```python
from build123d import *

# Parameters (mm, degrees)
F0_R     = 3.25
F0_R_2   = 1.85
F1_DEPTH = 4
F2_DEPTH = 4
F3_R     = 2.54


with BuildPart() as f1:
    # F0 (on Top) → F1 (new body)
    with BuildSketch(Plane.XY):
        with BuildLine():
            ThreePointArc((16, 9.294458), (9.088031, 9.088031), (9.294458, 16))
            Line((9.294458, 16), (-9.294458, 16))
            ThreePointArc((-9.294458, 16), (-8.114579, 14.394727), (-7.696788, 12.446788))
            ThreePointArc((-7.696788, 12.446788), (-10.760855, 8.006053), (-16, 9.294458))
            Line((-16, 9.294458), (-16, -9.294458))
            ThreePointArc((-16, -9.294458), (-10.760855, -8.006053), (-7.696788, -12.446788))
            ThreePointArc((-7.696788, -12.446788), (-8.114579, -14.394727), (-9.294458, -16))
            Line((-9.294458, -16), (9.294458, -16))
            ThreePointArc((9.294458, -16), (9.088031, -9.088031), (16, -9.294458))
            Line((16, -9.294458), (16, 9.294458))
        make_face()
        with Locations((-6.363961, -6.363961)):
            Circle(F0_R, mode=Mode.SUBTRACT)
        with Locations((6.363961, -6.363961)):
            Circle(F0_R, mode=Mode.SUBTRACT)
        with Locations((-6.363961, 6.363961)):
            Circle(F0_R, mode=Mode.SUBTRACT)
        with Locations((6.363961, 6.363961)):
            Circle(F0_R, mode=Mode.SUBTRACT)
        with BuildLine():
            ThreePointArc((-7.696788, 12.446788), (-8.114579, 14.394727), (-9.294458, 16))
            Line((-9.294458, 16), (-15.599119, 16))
            ThreePointArc((-15.599119, 16), (-15.805546, 15.805546), (-16, 15.599119))
            Line((-16, 15.599119), (-16, 9.294458))
            ThreePointArc((-16, 9.294458), (-10.760855, 8.006053), (-7.696788, 12.446788))
        make_face()
        with Locations((-12.446788, 12.446788)):
            Circle(F0_R_2, mode=Mode.SUBTRACT)
        with BuildLine():
            ThreePointArc((16, 15.599119), (15.805546, 15.805546), (15.599119, 16))
            Line((15.599119, 16), (9.294458, 16))
            ThreePointArc((9.294458, 16), (9.088031, 9.088031), (16, 9.294458))
            Line((16, 9.294458), (16, 15.599119))
        make_face()
        with Locations((12.446788, 12.446788)):
            Circle(F0_R_2, mode=Mode.SUBTRACT)
        with BuildLine():
            Line((16, -15.599119), (16, -9.294458))
            ThreePointArc((16, -9.294458), (9.088031, -9.088031), (9.294458, -16))
            Line((9.294458, -16), (15.599119, -16))
            ThreePointArc((15.599119, -16), (15.805546, -15.805546), (16, -15.599119))
        make_face()
        with Locations((12.446788, -12.446788)):
            Circle(F0_R_2, mode=Mode.SUBTRACT)
        with BuildLine():
            Line((-15.599119, -16), (-9.294458, -16))
            ThreePointArc((-9.294458, -16), (-8.114579, -14.394727), (-7.696788, -12.446788))
            ThreePointArc((-7.696788, -12.446788), (-10.760855, -8.006053), (-16, -9.294458))
            Line((-16, -9.294458), (-16, -15.599119))
            ThreePointArc((-16, -15.599119), (-15.805546, -15.805546), (-15.599119, -16))
        make_face()
        with Locations((-12.446788, -12.446788)):
            Circle(F0_R_2, mode=Mode.SUBTRACT)
        with BuildLine():
            ThreePointArc((-16, 15.599119), (-15.805546, 15.805546), (-15.599119, 16))
            Line((-15.599119, 16), (-16, 16))
            Line((-16, 16), (-16, 15.599119))
        make_face()
        with BuildLine():
            Line((16, 15.599119), (16, 16))
            Line((16, 16), (15.599119, 16))
            ThreePointArc((15.599119, 16), (15.805546, 15.805546), (16, 15.599119))
        make_face()
        with BuildLine():
            Line((16, -16), (16, -15.599119))
            ThreePointArc((16, -15.599119), (15.805546, -15.805546), (15.599119, -16))
            Line((15.599119, -16), (16, -16))
        make_face()
        with BuildLine():
            Line((-16, -16), (-15.599119, -16))
            ThreePointArc((-15.599119, -16), (-15.805546, -15.805546), (-16, -15.599119))
            Line((-16, -15.599119), (-16, -16))
        make_face()
    extrude(amount=F1_DEPTH)

    # F0 (on Top) → F2 (join)
    with BuildSketch(Plane.XY):
        with BuildLine():
            ThreePointArc((16, 9.294458), (9.088031, 9.088031), (9.294458, 16))
            Line((9.294458, 16), (-9.294458, 16))
            ThreePointArc((-9.294458, 16), (-8.114579, 14.394727), (-7.696788, 12.446788))
            ThreePointArc((-7.696788, 12.446788), (-10.760855, 8.006053), (-16, 9.294458))
            Line((-16, 9.294458), (-16, -9.294458))
            ThreePointArc((-16, -9.294458), (-10.760855, -8.006053), (-7.696788, -12.446788))
            ThreePointArc((-7.696788, -12.446788), (-8.114579, -14.394727), (-9.294458, -16))
            Line((-9.294458, -16), (9.294458, -16))
            ThreePointArc((9.294458, -16), (9.088031, -9.088031), (16, -9.294458))
            Line((16, -9.294458), (16, 9.294458))
        make_face()
        with Locations((-6.363961, -6.363961)):
            Circle(F0_R, mode=Mode.SUBTRACT)
        with Locations((6.363961, -6.363961)):
            Circle(F0_R, mode=Mode.SUBTRACT)
        with Locations((-6.363961, 6.363961)):
            Circle(F0_R, mode=Mode.SUBTRACT)
        with Locations((6.363961, 6.363961)):
            Circle(F0_R, mode=Mode.SUBTRACT)
        with Locations((-6.363961, -6.363961)):
            Circle(F0_R)
        with Locations((-6.363961, -6.363961)):
            Circle(F0_R_2, mode=Mode.SUBTRACT)
        with Locations((6.363961, -6.363961)):
            Circle(F0_R)
        with Locations((6.363961, -6.363961)):
            Circle(F0_R_2, mode=Mode.SUBTRACT)
        with Locations((6.363961, 6.363961)):
            Circle(F0_R)
        with Locations((6.363961, 6.363961)):
            Circle(F0_R_2, mode=Mode.SUBTRACT)
        with Locations((-6.363961, 6.363961)):
            Circle(F0_R)
        with Locations((-6.363961, 6.363961)):
            Circle(F0_R_2, mode=Mode.SUBTRACT)
    extrude(amount=-F2_DEPTH)

    # F3
    f3_edges = [f1.edges().sort_by_distance(p)[0] for p in [
        (16, 16, 2),
        (-16, 16, 2),
        (-16, -16, 2),
        (16, -16, 2),
    ]]
    fillet(f3_edges, radius=F3_R)


solid = f1.part
```
Design review of the part built by this model. Coordinates are the model's own, in mm. A direction names the side the tool comes from. Give positions to 0.01 mm unless a question says otherwise; leave off trailing zeros. Write each loop counter-clockwise with the first axis right and the second up, starting at its lowest first coordinate (ties: lowest second). Pieces come first, ordered by that corner, then holes. Notation, with made-up numbers: (55.25, 78.5) -> (80.25, 78.5) arc R16 cw to (80.25, 96.5) -> close; hole circle Ø8 at (-1.5, -7). An arc over 180 degrees is marked (long way). Answer in a Markdown table with one row per item.
(1) Consider section A-A (y = -12). State the section outline as (x, z) points, then the cut area to 3 significant figures.
Results:
| item | result |
|---|---|
| outline | (-16, 0) -> (-14.24, 0) -> (-14.24, 4) -> (-16, 4) -> close; (-10.65, 0) -> (-7.72, 0) -> (-7.72, -4) -> (7.72, -4) -> (7.72, 0) -> (10.65, 0) -> (10.65, 4) -> (-10.65, 4) -> close; (14.24, 0) -> (16, 0) -> (16, 4) -> (14.24, 4) -> close |
| area | 161 mm2 |
(2) Consider section B-B (x = 5). State the section outline as (y, z) points.
Results:
| item | result |
|---|---|
| outline | (-16, -4) -> (-7.61, -4) -> (-7.61, 0) -> (-9.31, 0) -> (-9.31, 4) -> (-16, 4) -> close; (-5.11, -4) -> (5.11, -4) -> (5.11, 0) -> (3.41, 0) -> (3.41, 4) -> (-3.41, 4) -> (-3.41, 0) -> (-5.11, 0) -> close; (7.61, -4) -> (16, -4) -> (16, 4) -> (9.31, 4) -> (9.31, 0) -> (7.61, 0) -> close |
(3) Clearance check with flat-ended pins moving along their axes: pin 1 (3 mm diameter, centred on x = -7, y = 5, fed in from +Z); pin 2 (2 mm diameter, centred on x = 6.36, y = 6.36, fed in from +Z); pin 3 (6.5 mm diameter, centred on x = -11.5, y = 13.5, fed in from -Z). State where each tip first meets the part, or that it passes through.
Results:
| item | result |
|---|---|
| pin 1 | z = 0 |
| pin 2 | through |
| pin 3 | z = 0 |
(4) To check wall thickness, follow probe 1 along Y at (x, z) = (9, -3.5); probe 2 along X at (y, z) = (12, 2.75); probe 3 along Y at (x, z) = (6, 0.5). State the ranges of each line that lie inside material, in increasing order.
Results:
| item | result |
|---|---|
| probe 1 | -16 to -15.72, -9.18 to 9.18, 15.72 to 16 |
| probe 2 | -16 to -14.24, -10.65 to 10.65, 14.24 to 16 |
| probe 3 | -16 to -9.59, -3.13 to 3.13, 9.59 to 16 |
(5) Consider section D-D (z = -1.25). State the section outline as (x, y) points.
Results:
| item | result |
|---|---|
| outline | (-16, -9.29) arc R4.75 cw to (-7.7, -12.45) arc R4.75 cw to (-9.29, -16) -> (9.29, -16) arc R4.75 cw (long way) to (16, -9.29) -> (16, 9.29) arc R4.75 cw (long way) to (9.29, 16) -> (-9.29, 16) arc R4.75 cw to (-7.7, 12.45) arc R4.75 cw to (-16, 9.29) -> close; hole circle Ø3.7 at (-6.36, -6.36); hole circle Ø3.7 at (-6.36, 6.36); hole circle Ø3.7 at (6.36, -6.36); hole circle Ø3.7 at (6.36, 6.36) |
(6) Mouldability with a two-part tool opening along Y and no side actions: class faces 4 (the cylindrical face through (-15.236, 15.276, 2.028)), 5 (the flat face through (0, 0, -4)), 6 (the cylindrical face through (-12.69, 14.28, 1.97)), 7 (the cylindrical face through (9.17, 9.01, -1.97)) as +Y half, -Y half, draft (parallel to the pull), parting line (faces both ways), or undercut.
Results:
| item | result |
|---|---|
| face 4 | +Y half |
| face 5 | draft |
| face 6 | undercut |
| face 7 | undercut |
(7) Consider section C-C (z = 2). Count the separate pieces of the cut face and the enclosed holes in it, then the cut area to 3 significant figures.
Results:
| item | result |
|---|---|
| separate pieces | 1 |
| enclosed holes | 8 |
| area | 843 mm2 |
(8) For faces 1 (the cylindrical face through (-9.61, 6.51, 1.97)), 2 (the cylindrical face through (-15.236, -15.276, 2.028)), 3 (the flat face through (11, -11, 0)), list the 3-axis set-ups (+Z, -Z, +X, -X, +Y, -Y) from which the entire face can be reached by the end or side of a thin tool; tool diameter is ignored.
Results:
| item | result |
|---|---|
| face 1 | +Z |
| face 2 | +Z, -Z, -X, -Y |
| face 3 | -Z |
